```python
from build123d import *

# Parameters (mm, degrees)
ESBO_O1_W                = 100
ESBO_O1_H                = 70
RESSALTO_EXTRUS_O1_DEPTH = 50
ESBO_O2_W                = 30
ESBO_O2_H                = 90
CORTE_EXTRUS_O1_DEPTH    = 239
ESBO_O3_R                = 4
CORTE_EXTRUS_O2_DEPTH    = 100
CORTE_EXTRUS_O3_REACH    = 133.909
ESBO_O4_W                = 60
ESBO_O4_H                = 80
FILETE2_R                = 2
FILETE3_R                = 2
ESBO_O5_R                = 15
CORTE_EXTRUS_O4_DEPTH    = 5
ESBO_O6_R                = 4
CORTE_EXTRUS_O7_DEPTH    = 239
PADR_OCIRCULAR1_COUNT    = 8


with BuildPart() as part:
    # Esboço1 → Ressalto-extrusão1 (new body)
    with BuildSketch(Plane(origin=(0, 0, 0), x_dir=(1, 0, 0), z_dir=(0, 1, 0))):
        with Locations((50, 35)):
            Rectangle(ESBO_O1_W, ESBO_O1_H)
    extrude(amount=-RESSALTO_EXTRUS_O1_DEPTH)

    # Esboço2 → Corte-extrusão1 (cut)
    with BuildSketch(Plane(origin=(0, 0, 0), x_dir=(0, 0, -1), z_dir=(1, 0, 0))):
        with Locations((35, -50)):
            Rectangle(ESBO_O2_W, ESBO_O2_H)
    extrude(amount=CORTE_EXTRUS_O1_DEPTH, mode=Mode.SUBTRACT)

    # Esboço3 → Corte-extrusão2 (cut)
    with BuildSketch(Plane(origin=(100, 0, 0), x_dir=(0, 0, -1), z_dir=(1, 0, 0))):
        with Locations((10, -25)):
            Circle(ESBO_O3_R)
        with Locations((60, -25)):
            Circle(ESBO_O3_R)
    extrude(amount=-CORTE_EXTRUS_O2_DEPTH, mode=Mode.SUBTRACT)

    # Corte-extrusão3: up to this face of the body (flat: up to its plane)
    corte_extrus_o3_end = Plane(part.part.faces().sort_by_distance((50, -25, -70))[0])
    # Esboço4 → Corte-extrusão3 (cut, up to the picked face)
    with BuildSketch(Plane.XY, mode=Mode.PRIVATE) as corte_extrus_o3_sk1:
        with Locations((50, -50)):
            Rectangle(ESBO_O4_W, ESBO_O4_H)
    corte_extrus_o3_tool1 = split(extrude(corte_extrus_o3_sk1.sketch, amount=-CORTE_EXTRUS_O3_REACH, mode=Mode.PRIVATE), bisect_by=corte_extrus_o3_end, keep=Keep.BOTH, mode=Mode.PRIVATE)
    add(corte_extrus_o3_tool1.solids().sort_by(Axis((50, -50, 0), (0, 0, -1)))[0], mode=Mode.SUBTRACT)

    # Filete2
    filete2_edges = [part.edges().sort_by_distance(p)[0] for p in [
        (0, -25, -70),
    ]]
    fillet(filete2_edges, radius=FILETE2_R)

    # Filete3
    filete3_edges = [part.edges().sort_by_distance(p)[0] for p in [
        (100, -25, -70),
        (100, -25, 0),
        (0, -25, 0),
    ]]
    fillet(filete3_edges, radius=FILETE3_R)

    # Esboço5 → Corte-extrusão4 (cut)
    with BuildSketch(Plane(origin=(0, 0, 0), x_dir=(1, 0, 0), z_dir=(0, 1, 0))):
        with Locations(Location((50, 35, 0), (0, 0, 270))):
            Circle(ESBO_O5_R)
    extrude(amount=-CORTE_EXTRUS_O4_DEPTH, mode=Mode.SUBTRACT)

    # Esboço6 → Corte-extrusão7 (cut)
    with BuildSketch(Plane(origin=(0, 0, 0), x_dir=(1, 0, 0), z_dir=(0, 1, 0))):
        with Locations(Location((50, 57.5, 0), (0, 0, 270))):
            Circle(ESBO_O6_R)
    corte_extrus_o7 = extrude(amount=-CORTE_EXTRUS_O7_DEPTH, mode=Mode.SUBTRACT)

    # PadrãoCircular1: Corte-extrusão7 ×8 about axis
    padr_ocircular1_axis = Axis((50, 0, -35), (0, 1, 0))
    for i in range(1, PADR_OCIRCULAR1_COUNT):
        add(corte_extrus_o7.rotate(padr_ocircular1_axis, i * 360 / PADR_OCIRCULAR1_COUNT), mode=Mode.SUBTRACT)


solid = part.part
```
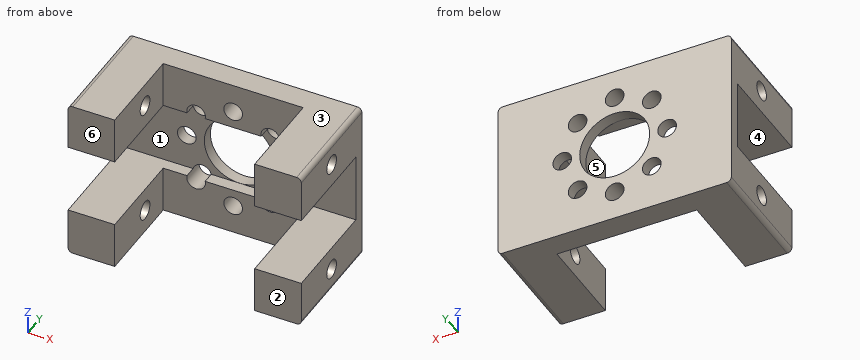
Design review of the part built by this model. Coordinates are the model's own, in mm. Face numbers are marked on the shaded views. A direction names the side the tool comes from. Give positions to 0.01 mm unless a question says otherwise; leave off trailing zeros. Write each loop counter-clockwise with the first axis right and the second up, starting at its lowest first coordinate (ties: lowest second). Pieces come first, ordered by that corner, then holes. Notation, with made-up numbers: (15.25, 11) - (74.25, 11) arc R17 cw to (74.25, 42) - close; hole circle Ø5 at (44, 58.25). An arc over 180 degrees is marked (long way). Return JSON: item names as keys, results as strings. Group by question number.
(1) Insertion check: pin 1 (15 mm diameter, centred on x = 29, z = -36.5, fed in from -Y); pin 2 (4 mm diameter, centred on x = 77, z = -55, fed in from -Y). Each pin has a flat end and moves straight along its axis. Give the tip position at first contact, or say it passes through.
(2) Machinability: for the marked faces 4, 5 and 6, which of the approach directions +Z, -Z, +X, -X, +Y, -Y give a long, thin tool a straight path to every point of the face, cutting with its end or side? Answer none if there is none.
(3) We need section D-D, the plane x = 86. Give the boundary of the cut face in (y, z).
(4) We need section C-C, the plane z = -35. Give the boundary of the cut face in (x, y), then the cut area to 3 significant figures.
(5) To check wall thickness, follow probe 1 along X at (y, z) = (-29, -62); probe 2 along Z at (x, y) = (87, -31); probe 3 along Y at (x, z) = (6, -10). State the ranges of each line that lie inside material, in increasing order.
(6) We need section B-B, the plane y = -19. Give the boundary of the cut face in (x, z), then the cut area to 3 significant figures.
(7) Mouldability with a two-part tool opening along Z and no side actions: class the marked faces 1, 2 and 3 as +Z half, -Z half, draft (parallel to the pull), parting line (faces both ways), or undercut.
(8) We need section A-A, the plane x = 27.5. Give the boundary of the cut face in (y, z), then the cut area to 3 significant figures.
Reported:
{
 "1": {"pin 1": "stops at y = -5", "pin 2": "stops at y = -10"},
 "2": {"face 4": "+X, -X, -Y", "face 5": "+Z, -Z, -Y", "face 6": "+Z, -Z, +X, -X, -Y"},
 "3": {"outline": "(-50, -70) - (0, -70) - (0, 0) - (-50, 0) - (-50, -20) - (-5, -20) - (-5, -50) - (-50, -50) - close; hole circle Ø8 at (-25, -60); hole circle Ø8 at (-25, -10)"},
 "4": {"outline": "(0, -5) - (23.5, -5) - (23.5, 0) - (0, 0) - close; (31.5, -5) - (35, -5) - (35, 0) - (31.5, 0) - close; (65, -5) - (68.5, -5) - (68.5, 0) - (65, 0) - close; (76.5, -5) - (100, -5) - (100, 0) - (76.5, 0) - close", "area": "270 mm2"},
 "5": {"probe 1": "x = 0 to 20, 80 to 100", "probe 2": "z = -70 to -50, -20 to 0", "probe 3": "y = -50 to -29, -21 to 0"},
 "6": {"outline": "(0, -68) arc R2 ccw to (2, -70) - (20, -70) - (20, -50) - (0, -50) - close; (0, -20) - (20, -20) - (20, 0) - (2, 0) arc R2 ccw to (0, -2) - close; (80, -70) - (98, -70) arc R2 ccw to (100, -68) - (100, -50) - (80, -50) - close; (80, -20) - (100, -20) - (100, -2) arc R2 ccw to (98, 0) - (80, 0) - close", "area": "1,600 mm2"},
 "7": {"face 1": "undercut", "face 2": "draft", "face 3": "+Z half"},
 "8": {"outline": "(-10, -70) - (0, -70) - (0, -39) - (-5, -39) - (-5, -50) - (-10, -50) - close; (-10, -20) - (-5, -20) - (-5, -31) - (0, -31) - (0, 0) - (-10, 0) - close", "area": "510 mm2"}
}
